The model under review builds one solid part; all positions refer to its coordinate system, in mm. Round coordinates to 2 decimals unless told otherwise and drop trailing zeros. Write each loop counter-clockwise with the first axis right and the second up, starting at its lowest first coordinate (ties: lowest second). Pieces come first, ordered by that corner, then holes. Notation, with made-up numbers: (84, 75.5) - (97, 75.5) arc R23 cw to (97, 86.5) - close; hole circle Ø1 at (4.25, 31). An arc over 180 degrees is marked (long way). Use one line per item in the form item = value.
Solid Edge part; units mm, degrees
sketch "Sketch1" plane through (0, 0, 0) normal (0, 0, 1) x (1, 0, 0)
  line L0 (0, 0) -> (50.8, 0)
  line L1 (50.8, 0) -> (50.8, 50.8)
  line L2 (50.8, 50.8) -> (0, 50.8)
  line L3 (0, 50.8) -> (0, 0)
extrude "Protrusion1" add sketch "Sketch1" along normal blind 3.175
hole "Hole_1" at (42.8625, 6.35, 3.175) direction (0, 0, -1) diameter 4.826 end up to next countersink diameter 9.525 countersink angle 82
hole "Hole1" at (7.9375, 6.35, 3.175) direction (0, 0, -1) diameter 4.826 end up to next countersink diameter 9.525 countersink angle 82
hole "Hole_2" at (25.4, 38.1, 3.175) direction (0, 0, -1) diameter 12.7 end up to next
chamfer "Chamfer_1" distance 6.35 angle 45 2 edges at (0, 50.8, 1.5875) (50.8, 50.8, 1.5875)
properties part number "CHAS-04" material "Aluminum, 1060"
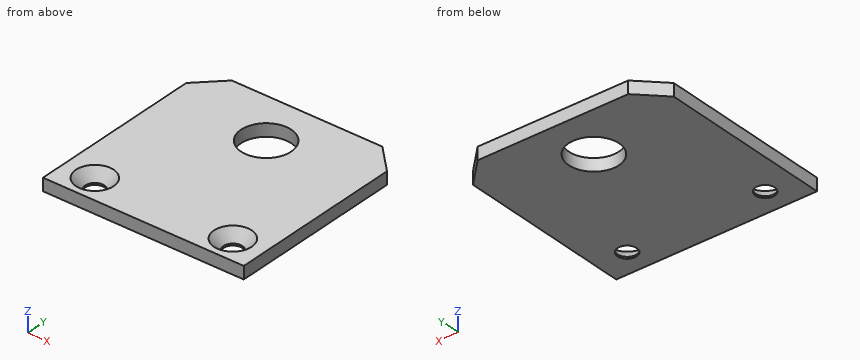
(1) Insertion check: P1, Ø4.5, axis at x = 7.94, y = 6.35, coming from the -Z side. The pin has a flat end and moves straight along its axis. Give the tip position at first contact, or say it passes through.
Geometry results:
P1 = through
(2) Add section B-B on y = 6.35. Write out the cut boundary in (x, z) (1 decimal), then the cut area to 3 significant figures.
Geometry results:
outline = (0, 0) - (5.5, 0) - (5.5, 0.5) - (3.2, 3.2) - (0, 3.2) - close; (10.4, 0) - (40.4, 0) - (40.4, 0.5) - (38.1, 3.2) - (12.7, 3.2) - (10.4, 0.5) - close; (45.3, 0) - (50.8, 0) - (50.8, 3.2) - (47.6, 3.2) - (45.3, 0.5) - close
area = 118 mm2
(3) Add section C-C on x = 25.4. Write out the cut boundary in (y, z) (3 decimals).
Geometry results:
outline = (0, 0) - (31.75, 0) - (31.75, 3.175) - (0, 3.175) - close; (44.45, 0) - (50.8, 0) - (50.8, 3.175) - (44.45, 3.175) - close
(4) Add section D-D on z = 2.05. Write out the cut boundary in (x, y), then the cut area to 3 significant figures.
Geometry results:
outline = (0, 0) - (50.8, 0) - (50.8, 44.45) - (44.45, 50.8) - (6.35, 50.8) - (0, 44.45) - close; hole circle Ø7.57 at (7.94, 6.35); hole circle Ø12.7 at (25.4, 38.1); hole circle Ø7.57 at (42.86, 6.35)
area = 2,320 mm2
(5) To check wall thickness, follow L1, parallel to X at y = 6.35, z = 0.45; L2, parallel to X at y = 38.1, z = 0.7; L3, parallel to Y at x = 25.4, z = 1.05. State the ranges of each line that lie inside material, in increasing order.
Geometry results:
L1 = 0 to 5.52, 10.35 to 40.45, 45.28 to 50.8
L2 = 0 to 19.05, 31.75 to 50.8
L3 = 0 to 31.75, 44.45 to 50.8
(6) Add section A-A on y = 38.1. Write out the cut boundary in (x, z) (3 decimals).
Geometry results:
outline = (0, 0) - (19.05, 0) - (19.05, 3.175) - (0, 3.175) - close; (31.75, 0) - (50.8, 0) - (50.8, 3.175) - (31.75, 3.175) - close
